```python
from build123d import *

# Parameters (mm, degrees)
SKETCH1_W                  = 130
SKETCH1_H                  = 150
BOSS_EXTRUDE1_DEPTH        = 3
F_10_0_10_DIAMETER_HOLE2_D = 10
F_14_0_14_DIAMETER_HOLE1_D = 14
F_5_0_5_DIAMETER_HOLE1_D   = 5
F_9_0_9_DIAMETER_HOLE1_D   = 9
F_5_0_5_DIAMETER_HOLE2_D   = 5
SKETCH15_W                 = 130
SKETCH15_H                 = 30
CUT_EXTRUDE1_DEPTH         = 199.517001791
SKETCH16_R                 = 2.35
CUT_EXTRUDE2_DEPTH         = 199.517001791


with BuildPart() as part:
    # Sketch1 → Boss-Extrude1 (new body)
    with BuildSketch(Plane(origin=(0, 0, 0), x_dir=(1, 0, 0), z_dir=(0, 1, 0))):
        with Locations((65, -75)):
            Rectangle(SKETCH1_W, SKETCH1_H)
    extrude(amount=BOSS_EXTRUDE1_DEPTH)

    # Ø10.0 (10) Diameter Hole2 (through all)
    with Locations(Plane(origin=(0, 3, 0), x_dir=(1, 0, 0), z_dir=(0, 1, 0))):
        with Locations((40, -128), (98, -128), (74, -66)):
            Hole(F_10_0_10_DIAMETER_HOLE2_D / 2)

    # Ø14.0 (14) Diameter Hole1 (through all)
    with Locations(Plane(origin=(0, 3, 0), x_dir=(1, 0, 0), z_dir=(0, 1, 0))):
        with Locations((16, -16), (114, -16)):
            Hole(F_14_0_14_DIAMETER_HOLE1_D / 2)

    # Ø5.0 (5) Diameter Hole1 (through all)
    with Locations(Plane(origin=(0, 3, 0), x_dir=(1, 0, 0), z_dir=(0, 1, 0))):
        with Locations((4.686291501, -27.313708499), (4.686291501, -4.686291501), (27.313708499, -4.686291501), (27.313708499, -27.313708499), (102.686291501, -27.313708499), (125.313708499, -27.313708499), (125.313708499, -4.686291501), (102.686291501, -4.686291501)):
            Hole(F_5_0_5_DIAMETER_HOLE1_D / 2)

    # Ø9.0 (9) Diameter Hole1 (through all)
    with Locations(Plane(origin=(0, 3, 0), x_dir=(1, 0, 0), z_dir=(0, 1, 0))):
        with Locations((65, -16)):
            Hole(F_9_0_9_DIAMETER_HOLE1_D / 2)

    # Ø5.0 (5) Diameter Hole2 (through all)
    with Locations(Plane(origin=(0, 3, 0), x_dir=(1, 0, 0), z_dir=(0, 1, 0))):
        with Locations((53.686291501, -27.313708499), (76.313708499, -27.313708499), (76.313708499, -4.686291501), (53.686291501, -4.686291501)):
            Hole(F_5_0_5_DIAMETER_HOLE2_D / 2)

    # Sketch15 → Cut-Extrude1 (cut, through all)
    with BuildSketch(Plane(origin=(0, 0, 0), x_dir=(1, 0, 0), z_dir=(0, 1, 0))):
        with Locations((65, -15)):
            Rectangle(SKETCH15_W, SKETCH15_H)
    extrude(amount=CUT_EXTRUDE1_DEPTH, mode=Mode.SUBTRACT)

    # Sketch16 → Cut-Extrude2 (cut, through all)
    with BuildSketch(Plane(origin=(0, 0, 0), x_dir=(1, 0, 0), z_dir=(0, 1, 0))):
        with Locations(Location((89.95, -37.25, 0), (0, 0, 90))):
            Circle(SKETCH16_R)
        with Locations(Location((118.05, -37.25, 0), (0, 0, 90))):
            Circle(SKETCH16_R)
        with Locations(Location((104, -40.25, 0), (0, 0, 90))):
            Circle(SKETCH16_R)
        with Locations(Location((11.95, -37.25, 0), (0, 0, 90))):
            Circle(SKETCH16_R)
        with Locations(Location((40.05, -37.25, 0), (0, 0, 90))):
            Circle(SKETCH16_R)
        with Locations(Location((26, -40.25, 0), (0, 0, 90))):
            Circle(SKETCH16_R)
    extrude(amount=CUT_EXTRUDE2_DEPTH, mode=Mode.SUBTRACT)


solid = part.part
```
The model under review builds one solid part; all positions refer to its coordinate system, in mm. Give positions to 0.01 mm unless a question says otherwise; leave off trailing zeros. Write each loop counter-clockwise with the first axis right and the second up, starting at its lowest first coordinate (ties: lowest second). Pieces come first, ordered by that corner, then holes.
(1) Consider section B-B, the plane y = 0.8. Give the number of separate pieces and of enclosed holes in the cut face, and give its area (3 significant figures).
(2) The part is to be moulded in two halves that separate along Z. For faces 1 (the cylindrical face through (102.018, 1.479, 38.987)), 2 (the cylindrical face through (11.24, 1.48, 35.01)), 3 (the flat face through (64, 3, 89)), 4 (the flat face through (64, 1, 30)), say which applies: released by +Z, released by -Z, zero draft, split by the parting line, or undercut.
(3) For P1, Ø9, axis at x = 74, z = 66, coming from the +Y side; P2, Ø11.5, axis at x = 40, z = 128, coming from the -Y side, all flat-tipped, find the tip position at first contact; note any pin that passes through.
(4) Consider section D-D, the plane z = 66. Give the boundary of the cut face in (x, y), and give its area (3 significant figures).
(5) To check wall thickness, follow L1, parallel to X at y = 1.1, z = 37.25; L2, parallel to X at y = 2.45, z = 128; L3, parallel to X at y = 0.3, z = 40.5. State the ranges of each line that lie inside material, in increasing order.
(6) Consider section C-C, the plane z = 128. Give the boundary of the cut face in (x, y), and give its area (3 significant figures).
(7) Consider section A-A, the plane x = 118.05. Give the boundary of the cut face in (y, z), and give its area (3 significant figures).
Returned:
1. separate pieces: 1
1. enclosed holes: 9
1. area: 15,300 mm2
2. face 1: undercut
2. face 2: undercut
2. face 3: zero draft
2. face 4: released by -Z
3. P1: passes through
3. P2: stops at y = 0
4. outline: (0, 0) - (69, 0) - (69, 3) - (0, 3) - close; (79, 0) - (130, 0) - (130, 3) - (79, 3) - close
4. area: 360 mm2
5. L1: x = 0 to 9.6, 14.3 to 37.7, 42.4 to 87.6, 92.3 to 115.7, 120.4 to 130
5. L2: x = 0 to 35, 45 to 93, 103 to 130
5. L3: x = 0 to 23.66, 28.34 to 101.66, 106.34 to 130
6. outline: (0, 0) - (35, 0) - (35, 3) - (0, 3) - close; (45, 0) - (93, 0) - (93, 3) - (45, 3) - close; (103, 0) - (130, 0) - (130, 3) - (103, 3) - close
6. area: 330 mm2
7. outline: (0, 30) - (3, 30) - (3, 34.9) - (0, 34.9) - close; (0, 39.6) - (3, 39.6) - (3, 150) - (0, 150) - close
7. area: 346 mm2
